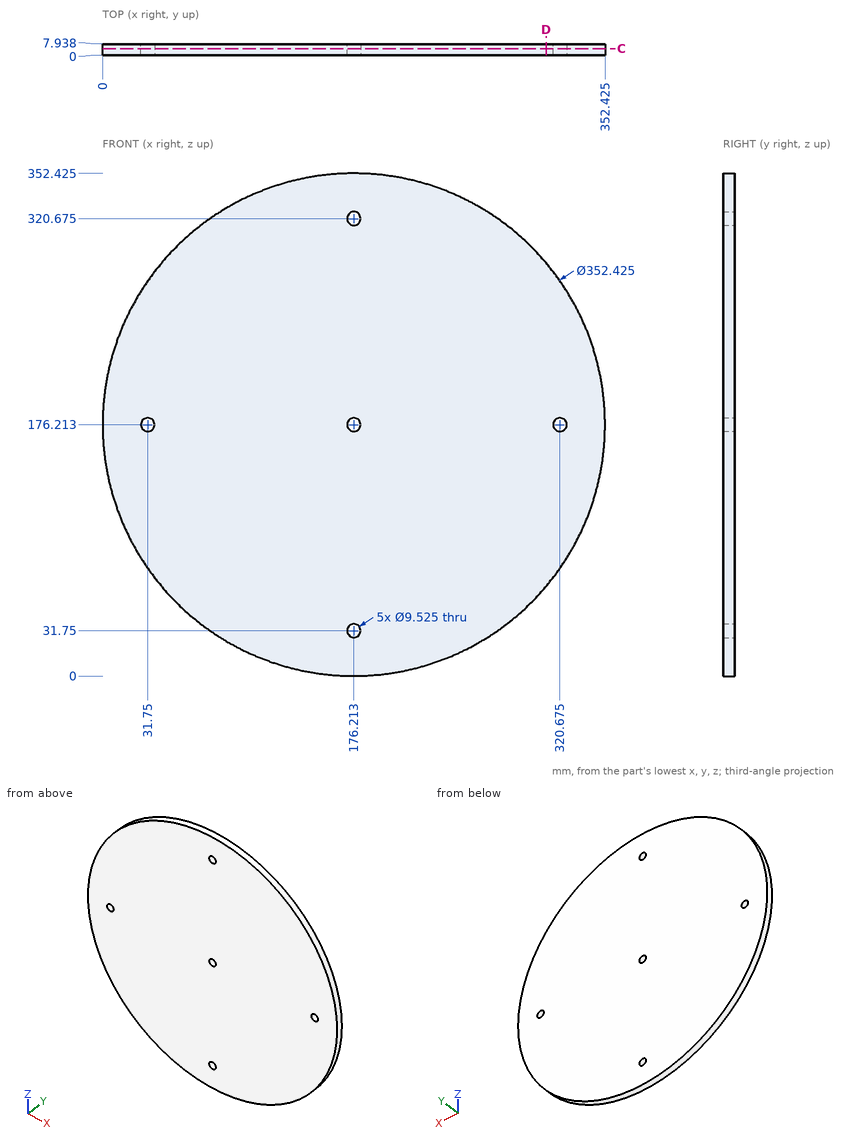
Could you check a few things on this drawing? It's one solid part, dimensions in mm from its lowest x, y, z. Give positions to 0.01 mm unless a question says otherwise; leave off trailing zeros. Order: outer loops, then holes, each group sorted by start corner. A loop starts at its lowest first (then second) coordinate and runs counter-clockwise, first axis right, second up. Notation, with made-up numbers: (85, -26) - (113, -26) arc R25 cw to (113, -6) - close; hole circle Ø10 at (74, 48.5). An arc over 180 degrees is marked (long way). One line per item, written item: value. Start each with the question number.
1. Imagine slicing it at D-D on x = 311. List the corners of the cut face in (y, z) for me, plus the area to 3 significant figures.
2. If I drill on probe 1 along Z at (x, y) = (178, 1) (1 decimal); probe 2 along X at (y, z) = (4.75, 32.5) (1 decimal); probe 3 along X at (y, z) = (1, 126.5), over which ranges is the centre line in solid material (lowest first)?
3. For P1, Ø2, axis at y = 1.5, z = 293, coming from the +X side (1 decimal); P2, Ø2, axis at y = 1.5, z = 266, coming from the +X side; P3, Ø7.5, axis at x = 31.75, z = 176.21, coming from the -Y side; P4, Ø1, axis at y = 5.5, z = 307, coming from the +X side (1 decimal), each with a flat end and sliding along its axis, tell me the tip position at first contact or that it passes through.
4. Imagine slicing it at C-C on y = 4.75. Give the number of separate pieces and of enclosed holes in the cut face, plus the area to 3 significant figures.
Values:
1. outline: (0, 62.71) - (7.94, 62.71) - (7.94, 289.72) - (0, 289.72) - close
1. area: 1,800 mm²
2. probe 1: 0 to 27.3, 36.2 to 171.8, 180.6 to 316.3, 325.1 to 352.4
2. probe 2: 74.2 to 171.5, 180.9 to 278.2
2. probe 3: 7.16 to 345.27
3. P1: x = 309
3. P2: x = 328.42
3. P3: through
3. P4: x = 294.9
4. separate pieces: 1
4. enclosed holes: 5
4. area: 97,200 mm²
